Autodesk Inventor part; units mm, degrees
ref_plane "YZ Plane" through (0, 0, 0) normal (1, 0, 0) x (0, 1, 0)
ref_plane "XZ Plane" through (0, 0, 0) normal (0, 1, 0) x (-1, 0, 0)
ref_plane "XY Plane" through (0, 0, 0) normal (0, 0, 1) x (1, 0, 0)
sketch "Sketch1" plane through (0, 0, 0) normal (0, 0, 1) x (1, 0, 0)
  circle A0 centre (0, 0) radius 115
  circle A1 centre (0, 0) radius 220
  dimension "d22" = 230
  dimension "d23" = 440
extrude "Plate1" add sketch "Sketch1" along normal blind 4
sketch "Sketch5" plane through (0, 0, 4) normal (0, 0, 1) x (1, 0, 0)
  circle A0 centre (0, 200) radius 11
  circle A1 centre (0, 0) radius 200 construction
  dimension "d25" = 400
  dimension "d24" = 22
extrude "Cut1" cut sketch "Sketch5" against normal blind 4
pattern_circular "Circular Pattern1" count 12 over 360 about axis through (0, 0, 0) along (0, 0, 1) of "Cut1"
equation "\"d26\" = Thickness"
equation "\"d2\" = Thickness"
equation "\"BendReliefWidth\" = Thickness"
equation "\"BendReliefDepth\" = 0.5 * Thickness"
equation "\"CornerReliefSize\" = 4 * Thickness"
equation "\"MinimumRemnant\" = 2 * Thickness"
equation "\"TransitionRadius\" = BendRadius"
equation "\"JacobiRadiusSize\" = BendRadius"
equation "\"GapSize\" = Thickness"
properties part number "TKS 3212 flange separator" material "Stainless Steel"
The model under review builds one solid part; all positions refer to its coordinate system, in mm. Coordinates: 2 decimals unless noted, no trailing zeros. Write each loop counter-clockwise with the first axis right and the second up, starting at its lowest first coordinate (ties: lowest second). Pieces come first, ordered by that corner, then holes. Notation, with made-up numbers: (-16, 26) -> (22, 26) arc R24 ccw to (22, 40) -> close; hole circle Ø10 at (50, 75). An arc over 180 degrees is marked (long way). Answer in a Markdown table with one row per item.
1. Draft analysis for pull direction X (two halves, no side actions). For faces 1 (the cylindrical face through (1.432, -210.906, 2.028)), 2 (the flat face through (95, -95, 0)), 3 (the cylindrical face through (-47.69, 214.77, 1.97)), state which applies: +X half, -X half, draft (parallel to the pull), parting line (faces both ways), or undercut.
Answers below:
| item | result |
|---|---|
| face 1 | undercut |
| face 2 | draft |
| face 3 | parting line |
2. We need section C-C, the plane y = 64.5. State the section outline as (x, z) points.
Answers below:
| item | result |
|---|---|
| outline | (-210.33, 0) -> (-95.21, 0) -> (-95.21, 4) -> (-210.33, 4) -> close; (95.21, 0) -> (210.33, 0) -> (210.33, 4) -> (95.21, 4) -> close |
3. We need section A-A, the plane y = 0. State the section outline as (x, z) points, and give its area (3 significant figures).
Answers below:
| item | result |
|---|---|
| outline | (-220, 0) -> (-211, 0) -> (-211, 4) -> (-220, 4) -> close; (-189, 0) -> (-115, 0) -> (-115, 4) -> (-189, 4) -> close; (115, 0) -> (189, 0) -> (189, 4) -> (115, 4) -> close; (211, 0) -> (220, 0) -> (220, 4) -> (211, 4) -> close |
| area | 664 mm^2 |
4. We need section D-D, the plane x = 104.5. State the section outline as (y, z) points.
Answers below:
| item | result |
|---|---|
| outline | (-193.6, 0) -> (-183.24, 0) -> (-183.24, 4) -> (-193.6, 4) -> close; (-163.17, 0) -> (-48.01, 0) -> (-48.01, 4) -> (-163.17, 4) -> close; (48.01, 0) -> (163.17, 0) -> (163.17, 4) -> (48.01, 4) -> close; (183.24, 0) -> (193.6, 0) -> (193.6, 4) -> (183.24, 4) -> close |
5. We need section B-B, the plane x = -21. State the section outline as (y, z) points.
Answers below:
| item | result |
|---|---|
| outline | (-219, 0) -> (-113.07, 0) -> (-113.07, 4) -> (-219, 4) -> close; (113.07, 0) -> (219, 0) -> (219, 4) -> (113.07, 4) -> close |
6. Wall thickness on probe 1 along Y at (x, z) = (2.5, 2.8); probe 2 along X at (y, z) = (169, 1.25); probe 3 along X at (y, z) = (-178.5, 0.9): over which ranges is each line inside the solid? List them lowest first. Write a range as [from, to].
Answers below:
| item | result |
|---|---|
| probe 1 | y = [-219.99, -210.71], [-189.29, -114.97], [114.97, 189.29], [210.71, 219.99] |
| probe 2 | x = [-140.85, -110.16], [-89.84, 89.84], [110.16, 140.85] |
| probe 3 | x = [-128.6, -109.64], [-90.36, 90.36], [109.64, 128.6] |
7. Clearance check with a flat-ended pin moving along its axis: pin 1 Ø1 at (y, z) = (158, 3.5) entering from +X. State where the tip first meets the part, or that it passes through.
Answers below:
| item | result |
|---|---|
| pin 1 | stops at x = 153.6 |
